Build history of the part. All positions in model axes, mm. Face numbers are marked on the shaded views. Give positions to 0.01 mm unless a question says otherwise; leave off trailing zeros. Order: outer loops, then holes, each group sorted by start corner. A loop starts at its lowest first (then second) coordinate and runs counter-clockwise, first axis right, second up. Notation, with made-up numbers: (55, -2) - (66, -2) arc R27 ccw to (66, 27) - close; hole circle Ø8 at (-29, 11). An arc over 180 degrees is marked (long way). One line per item, written item: value.
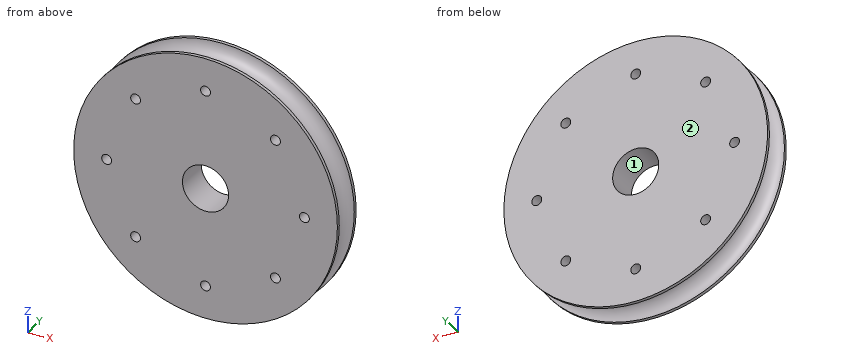
```python
from build123d import *

# Parameters (mm, degrees)
SKETCH1_R           = 20
SKETCH1_R_2         = 3.5
BOSS_EXTRUDE1_DEPTH = 5
SKETCH3_R           = 0.75
CUT_EXTRUDE1_DEPTH  = 6


with BuildPart() as part:
    # Sketch1 → Boss-Extrude1 (new body)
    with BuildSketch(Plane(origin=(0, 0, 0), x_dir=(1, 0, 0), z_dir=(0, 1, 0))):
        Circle(SKETCH1_R)
        Circle(SKETCH1_R_2, mode=Mode.SUBTRACT)
    extrude(amount=BOSS_EXTRUDE1_DEPTH)

    # Sketch2 → Cut-Revolve1 (revolve, cut)
    with BuildSketch(Plane.XY):
        with BuildLine():
            Line((-20, 0.5), (-20, 4.5))
            ThreePointArc((-20, 4.5), (-18, 2.5), (-20, 0.5))
        make_face()
    revolve(axis=Axis((0, 0, 0), (0, 1, 0)), mode=Mode.SUBTRACT)

    # Sketch3 → Cut-Extrude1 (cut, through all)
    with BuildSketch(Plane(origin=(0, 0, 0), x_dir=(1, 0, 0), z_dir=(0, 1, 0))):
        with Locations((0, -15)):
            Circle(SKETCH3_R)
        with Locations((-10.606601718, -10.606601718)):
            Circle(SKETCH3_R)
        with Locations((-15, 0)):
            Circle(SKETCH3_R)
        with Locations((-10.606601718, 10.606601718)):
            Circle(SKETCH3_R)
        with Locations((0, 15)):
            Circle(SKETCH3_R)
        with Locations((10.606601718, 10.606601718)):
            Circle(SKETCH3_R)
        with Locations((15, 0)):
            Circle(SKETCH3_R)
        with Locations((10.606601718, -10.606601718)):
            Circle(SKETCH3_R)
    extrude(amount=CUT_EXTRUDE1_DEPTH, mode=Mode.SUBTRACT)


solid = part.part
```
(1) Slice it at B-B, the plane y = 2.95. Count the separate pieces of the cut face and the enclosed holes in it, and give its area (3 significant figures).
Completed:
separate pieces: 1
enclosed holes: 9
area: 971 mm²
(2) Slice it at A-A, the plane x = 0. Give the cut face in (y, z).
Completed:
outline: (0, -20) - (0.5, -20) arc R2 cw to (4.5, -20) - (5, -20) - (5, -15.75) - (0, -15.75) - close; (0, -14.25) - (5, -14.25) - (5, -3.5) - (0, -3.5) - close; (0, 3.5) - (5, 3.5) - (5, 14.25) - (0, 14.25) - close; (0, 15.75) - (5, 15.75) - (5, 20) - (4.5, 20) arc R2 cw to (0.5, 20) - (0, 20) - close
(3) Pull direction Z, two halves, no side cores. Call the marked faces 1 and 2: +Z half, -Z half, draft (parallel to the pull), parting line (faces both ways), or undercut.
Completed:
face 1: undercut
face 2: draft
(4) Pin check, flat tips, straight feed: P1, Ø2, axis at x = -5.5, y = 2.5, coming from the -Z side; P2, Ø1.5, axis at x = -2.5, y = 1.5, coming from the +Z side; P3, Ø2, axis at x = 4, y = 4, coming from the -Z side. Stop position of each tip, or through.
Completed:
P1: z = -17.5
P2: z = 18.87
P3: z = -19.75
(5) Drill centre lines: line 1 (X direction, y = 2.8, z = 10); line 2 (Z direction, x = 0, y = 2.85); line 3 (Z direction, x = 0, y = 3.45). Where is each one in solid material? Low to high.
Completed:
line 1: -14.99 to -11.05, -10.17 to 10.17, 11.05 to 14.99
line 2: -18.03 to -15.75, -14.25 to -3.5, 3.5 to 14.25, 15.75 to 18.03
line 3: -18.24 to -15.75, -14.25 to -3.5, 3.5 to 14.25, 15.75 to 18.24
